Autodesk Inventor part; units mm, degrees
ref_plane "YZ Plane" through (0, 0, 0) normal (1, 0, 0) x (0, 1, 0)
ref_plane "XZ Plane" through (0, 0, 0) normal (0, 1, 0) x (-1, 0, 0)
ref_plane "XY Plane" through (0, 0, 0) normal (0, 0, 1) x (1, 0, 0)
sketch "Sketch1" plane through (0, 0, 0) normal (0, 1, 0) x (-1, 0, 0)
  line L0 (-10, 5) -> (10, 5)
  line L1 (10, 5) -> (10, -5)
  line L2 (10, -5) -> (-10, -5)
  line L3 (-10, -5) -> (-10, 5)
  line L4 (-10, 5) -> (10, -5) construction
  line L5 (10, 5) -> (-10, -5) construction
  point P0 (0, 0)
  dimension "d0" = 20
  dimension "d1" = 10
extrude "Extrusion1" add sketch "Sketch1" along normal blind 5
sketch "Sketch7" plane through (0, 5, 0) normal (0, 1, 0) x (1, 0, 0)
  line L0 (10, -20) -> (-10, -20)
  line L1 (-10, -20) -> (-10, 20)
  line L2 (-10, 20) -> (10, 20)
  line L3 (10, 20) -> (10, -20)
  line L4 (10, -20) -> (-10, 20) construction
  line L5 (-10, -20) -> (10, 20) construction
  point P0 (0, 0)
  dimension "d26" = 40
extrude "Extrusion4" add sketch "Sketch7" along normal blind 5
sketch "Sketch8" plane through (0, 10, 0) normal (0, 1, 0) x (1, 0, 0)
  line L0 (10, 20) -> (-10, 20)
  line L1 (10, 5) -> (10, 20)
  line L2 (-10, 20) -> (10, 20)
  line L3 (10, 20) -> (10, 15)
  line L4 (10, 15) -> (-10, 15)
  line L5 (-10, 15) -> (-10, 20)
  point P0 (0, 0)
  dimension "d29" = 5
extrude "Extrusion5" add sketch "Sketch8" along normal blind 120
sketch "Sketch9" plane through (0, 10, 0) normal (0, 1, 0) x (1, 0, 0)
  line L0 (10, 15) -> (-10, 15)
  line L1 (10, -20) -> (10, 15)
  line L2 (-10, 15) -> (10, 15)
  line L3 (10, 15) -> (10, 5)
  line L4 (10, 5) -> (-10, 5)
  line L5 (-10, 5) -> (-10, 15)
  point P0 (0, 0)
  dimension "d32" = 10
extrude "Extrusion6" add sketch "Sketch9" along normal blind 50
chamfer "Chamfer1" distance 10 distance2 50 1 edges at (0, 60, -5) measured on face at (-3.3333, 60, -11.6667)
sketch "Sketch10" plane through (0, 10, 0) normal (0, 1, 0) x (1, 0, 0)
  point P0 (0, 0)
  point P1 (0, 0)
hole "Hole3" at (0, 10, 0) direction (0, -1, 0) diameter 3.5 depth 10
sketch "Sketch11" plane through (-10, 130, -15) normal (0, 0, 1) x (1, 0, 0)
  line L0 (2.5, -8.75) -> (17.5, -8.75)
  line L1 (17.5, -8.75) -> (17.5, -5.25)
  line L2 (17.5, -5.25) -> (2.5, -5.25)
  line L3 (2.5, -5.25) -> (2.5, -8.75)
  line L4 (2.5, -8.75) -> (17.5, -5.25) construction
  line L5 (17.5, -8.75) -> (2.5, -5.25) construction
  line L6 (2.5, -10.25) -> (17.5, -10.25)
  line L7 (17.5, -10.25) -> (17.5, -13.75)
  line L8 (17.5, -13.75) -> (2.5, -13.75)
  line L9 (2.5, -13.75) -> (2.5, -10.25)
  line L10 (2.5, -10.25) -> (17.5, -13.75) construction
  line L11 (17.5, -10.25) -> (2.5, -13.75) construction
  line L12 (2.5, -15.25) -> (17.5, -15.25)
  line L13 (17.5, -15.25) -> (17.5, -18.75)
  line L14 (17.5, -18.75) -> (2.5, -18.75)
  line L15 (2.5, -18.75) -> (2.5, -15.25)
  line L16 (2.5, -15.25) -> (17.5, -18.75) construction
  line L17 (17.5, -15.25) -> (2.5, -18.75) construction
  line L18 (2.5, -23.75) -> (17.5, -23.75)
  line L19 (17.5, -23.75) -> (17.5, -20.25)
  line L20 (17.5, -20.25) -> (2.5, -20.25)
  line L21 (2.5, -20.25) -> (2.5, -23.75)
  line L22 (2.5, -23.75) -> (17.5, -20.25) construction
  line L23 (17.5, -23.75) -> (2.5, -20.25) construction
  line L24 (2.5, -34.15) -> (17.5, -34.15)
  line L25 (17.5, -34.15) -> (17.5, -30.65)
  line L26 (17.5, -30.65) -> (2.5, -30.65)
  line L27 (2.5, -30.65) -> (2.5, -34.15)
  line L28 (2.5, -34.15) -> (17.5, -30.65) construction
  line L29 (17.5, -34.15) -> (2.5, -30.65) construction
  line L30 (2.5, -39.15) -> (17.5, -39.15)
  line L31 (17.5, -39.15) -> (17.5, -35.65)
  line L32 (17.5, -35.65) -> (2.5, -35.65)
  line L33 (2.5, -35.65) -> (2.5, -39.15)
  line L34 (2.5, -39.15) -> (17.5, -35.65) construction
  line L35 (17.5, -39.15) -> (2.5, -35.65) construction
  line L36 (2.5, -44.15) -> (17.5, -44.15)
  line L37 (17.5, -44.15) -> (17.5, -40.65)
  line L38 (17.5, -40.65) -> (2.5, -40.65)
  line L39 (2.5, -40.65) -> (2.5, -44.15)
  line L40 (2.5, -44.15) -> (17.5, -40.65) construction
  line L41 (17.5, -44.15) -> (2.5, -40.65) construction
  line L42 (2.5, -49.15) -> (17.5, -49.15)
  line L43 (17.5, -49.15) -> (17.5, -45.65)
  line L44 (17.5, -45.65) -> (2.5, -45.65)
  line L45 (2.5, -45.65) -> (2.5, -49.15)
  line L46 (2.5, -49.15) -> (17.5, -45.65) construction
  line L47 (17.5, -49.15) -> (2.5, -45.65) construction
  point P0 (10, -130)
  point P1 (10, -7)
  point P2 (10, -32.4)
  point P3 (10, -12)
  point P4 (10, -37.4)
  point P5 (10, -17)
  point P6 (10, -42.4)
  point P7 (10, -22)
  point P8 (10, -47.4)
  dimension "d52" = 15
  dimension "d53" = 3.5
  dimension "d54" = 3.5
  dimension "d55" = 3.5
  dimension "d56" = 3.5
  dimension "d57" = 3.5
  dimension "d58" = 3.5
  dimension "d59" = 3.5
  dimension "d60" = 3.5
extrude "Extrusion7" cut sketch "Sketch11" against normal through all
properties part number "Indu_Holder"
For this review, take the finished solid that the model builds, in its own axes (mm). A direction names the side the tool comes from. Round coordinates to 2 decimals unless told otherwise and drop trailing zeros. Loops run counter-clockwise (first coordinate to the right, second up) from the corner with the lowest first, then second, coordinate; pieces in that order, holes last. Notation, with made-up numbers: (-34.75, 22.5) - (-11.75, 22.5) arc R34 ccw to (-11.75, 52.5) - close; hole circle Ø2 at (3, 85). An arc over 180 degrees is marked (long way). Use one line per item in the form item = value.
1) We need section D-D on y = 64. Write out the cut boundary in (x, z).
Solutions:
outline = (-10, -20) - (10, -20) - (10, -15) - (-10, -15) - close
2) Mouldability with a two-part tool opening along Z and no side actions: class faces 5 (the face through (-7.5, 98, -17)), 6 (the face through (0.67, 4.93, 1.617)), 7 (the face through (0, 7, 20)) as pulls with the +Z half, pulls with the -Z half, needs draft (parallel to the pull), parting line crosses it, or undercut.
Solutions:
face_5 = needs draft
face_6 = undercut
face_7 = pulls with the +Z half
3) We need section B-B on y = 113.5. Write out the cut boundary in (x, z), then the cut area to 3 significant figures.
Solutions:
outline = (-10, -20) - (-7.5, -20) - (-7.5, -15) - (-10, -15) - close; (7.5, -20) - (10, -20) - (10, -15) - (7.5, -15) - close
area = 25.0 mm2
4) We need section C-C on x = -3.75. State how many separate pieces and enclosed holes the cut face has, then the cut area to 3 significant figures.
Solutions:
separate_pieces = 9
enclosed_holes = 0
area = 960 mm2
5) Clearance check with flat-ended pins moving along their axes: P1, Ø2, axis at x = 0, z = 0, coming from the +Y side; P2, Ø10, axis at x = 2.5, y = 22, coming from the +Z side; P3, Ø4, axis at x = 3, z = -17.5, coming from the -Y side; P4, Ø12, axis at x = 0, z = -10, coming from the -Y side. State where each tip first meets the part, or that it passes through.
Solutions:
P1 = through
P2 = -6.4
P3 = 5
P4 = 0
6) Wall thickness on probe 1 along X at (y, z) = (6.25, 0); probe 2 along Z at (x, y) = (0, 3.75); probe 3 along Z at (x, y) = (0, 8): over which ranges is each line inside the solid? List them lowest first.
Solutions:
probe_1 = -10 to -1.75, 1.75 to 10
probe_2 = -5 to -1.75, 1.75 to 5
probe_3 = -20 to -1.75, 1.75 to 20
7) We need section A-A on z = 0. Write out the cut boundary in (x, y), then the cut area to 3 significant figures.
Solutions:
outline = (-10, 0) - (-1.75, 0) - (-1.75, 10) - (-10, 10) - close; (1.75, 0) - (10, 0) - (10, 10) - (1.75, 10) - close
area = 165 mm2
8) Tool access review of faces 1 (the face through (7.5, 123, -17)), 2 (the face through (0, 5, -13)), 3 (the face through (0, 5, 12)), 4 (the face through (0, 0, 2)): name each direction out of +Z, -Z, +X, -X, +Y, -Y from which nothing blocks a thin tool from reaching the whole face with its end or side.
Solutions:
face_1 = +Z, -Z
face_2 = -Z, +X, -X, -Y
face_3 = +Z, +X, -X, -Y
face_4 = +Z, -Z, +X, -X, -Y
